from build123d import *

# Parameters (mm, degrees)
BOSS_EXTRUDE1_DEPTH = 1.016


with BuildPart() as part:
    # Sketch1 → Boss-Extrude1 (new body)
    with BuildSketch(Plane.XY):
        with BuildLine():
            Line((-102.690520384, 151.318398839), (-130.138661403, 140.228630017))
            ThreePointArc((-130.138661403, 140.228630017), (-139.028894565, 132.36321613), (-140.988038021, 120.655836484))
            Line((-140.988038021, 120.655836484), (-122.083041186, 13.440271634))
            ThreePointArc((-122.083041186, 13.440271634), (-118.354836941, 5.294136523), (-111.127725304, 0))
            Line((-111.127725304, 0), (111.127725304, 0))
            ThreePointArc((111.127725304, 0), (118.354836941, 5.294136523), (122.083041186, 13.440271634))
            Line((122.083041186, 13.440271634), (140.988038021, 120.655836484))
            ThreePointArc((140.988038021, 120.655836484), (139.028894565, 132.36321613), (130.138661403, 140.228630017))
            Line((130.138661403, 140.228630017), (102.690520384, 151.318398839))
            ThreePointArc((102.690520384, 151.318398839), (92.216863272, 163.055161588), (95.154949405, 178.50885833))
            ThreePointArc((95.154949405, 178.50885833), (122.006673364, 200.829543277), (155.995276019, 208.829727371))
            Line((155.995276019, 208.829727371), (246.294572316, 208.829727371))
            ThreePointArc((246.294572316, 208.829727371), (251.682725989, 211.061573699), (253.914572316, 216.449727371))
            Line((253.914572316, 216.449727371), (253.914572316, 220.98))
            ThreePointArc((253.914572316, 220.98), (251.682725989, 226.368153673), (246.294572316, 228.6))
            Line((246.294572316, 228.6), (47.442005026, 228.6))
            ThreePointArc((47.442005026, 228.6), (20.63063365, 239.70563365), (9.525, 266.517005026))
            Line((9.525, 266.517005026), (9.525, 609.6))
            Line((9.525, 609.6), (-9.525, 609.6))
            Line((-9.525, 609.6), (-9.525, 266.517005026))
            ThreePointArc((-9.525, 266.517005026), (-20.63063365, 239.70563365), (-47.442005026, 228.6))
            Line((-47.442005026, 228.6), (-551.265427684, 228.6))
            ThreePointArc((-551.265427684, 228.6), (-556.653581357, 226.368153673), (-558.885427684, 220.98))
            Line((-558.885427684, 220.98), (-558.885427684, 216.449727371))
            ThreePointArc((-558.885427684, 216.449727371), (-556.653581357, 211.061573699), (-551.265427684, 208.829727371))
            Line((-551.265427684, 208.829727371), (-155.995276019, 208.829727371))
            ThreePointArc((-155.995276019, 208.829727371), (-122.006673364, 200.829543277), (-95.154949405, 178.50885833))
            ThreePointArc((-95.154949405, 178.50885833), (-92.216863272, 163.055161588), (-102.690520384, 151.318398839))
        make_face()
    extrude(amount=BOSS_EXTRUDE1_DEPTH)


solid = part.part
Verification items for the finished model (mm, model axes). A direction names the side the tool comes from. Coordinates: 2 decimals unless noted, no trailing zeros. Order: outer loops, then holes, each group sorted by start corner. A loop starts at its lowest first (then second) coordinate and runs counter-clockwise, first axis right, second up.
1. Release check for a two-part mould opening along Y. For faces 3 (the face through (131.403, 66.298, 0.501)), 4 (the face through (20.93, 239.41, 0.5)), 5 (the face through (-34, 171, 1.016)), 6 (the face through (-122.45, 201.05, 0.5)) record: +Y half, -Y half, draft (parallel to the pull), parting line (faces both ways), or undercut.
Results found:
face 3: -Y half
face 4: +Y half
face 5: draft
face 6: undercut
2. Sectioned sample at A-A, the plane z = 0.25. Record the cut outline in (x, y) (3 decimals), and give its area (3 significant figures).
Results found:
outline: (-558.885, 216.45) arc R7.62 ccw to (-551.265, 208.83) - (-155.995, 208.83) arc R76.2 cw to (-95.155, 178.509) arc R17.78 cw to (-102.691, 151.318) - (-130.139, 140.229) arc R17.78 ccw to (-140.988, 120.656) - (-122.083, 13.44) arc R17.78 ccw to (-111.128, 0) - (111.128, 0) arc R17.78 ccw to (122.083, 13.44) - (140.988, 120.656) arc R17.78 ccw to (130.139, 140.229) - (102.691, 151.318) arc R17.78 cw to (95.155, 178.509) arc R76.2 cw to (155.995, 208.83) - (246.295, 208.83) arc R7.62 ccw to (253.915, 216.45) - (253.915, 220.98) arc R7.62 ccw to (246.295, 228.6) - (47.442, 228.6) arc R37.917 cw to (9.525, 266.517) - (9.525, 609.6) - (-9.525, 609.6) - (-9.525, 266.517) arc R37.917 cw to (-47.442, 228.6) - (-551.265, 228.6) arc R7.62 ccw to (-558.885, 220.98) - close
area: 75,300 mm2
3. Go/stop test with a flat-tipped pin: pin 1 Ø0.5 at (x, z) = (202.5, 0.5) entering from -Y. Record where the tip stops, or that it passes through.
Results found:
pin 1: stops at y = 208.83
4. Sectioned sample at C-C, the plane y = 458.5. Record the cut outline in (x, z) (3 decimals).
Results found:
outline: (-9.525, 0) - (9.525, 0) - (9.525, 1.016) - (-9.525, 1.016) - close
5. Scan lines: line 1 (Y direction, x = -292.5, z = 0.85); line 2 (X direction, y = 380.5, z = 0.35) (3 decimals); line 3 (Y direction, x = -89.5, z = 0.25). Record each from-to range of solid material in increasing order.
Results found:
line 1: y = 208.83 to 228.6
line 2: x = -9.525 to 9.525
line 3: y = 0 to 228.6
6. Sectioned sample at B-B, the plane x = -249. Record the cut outline in (y, z), and give its area (3 significant figures).
Results found:
outline: (208.83, 0) - (228.6, 0) - (228.6, 1.02) - (208.83, 1.02) - close
area: 20.1 mm2
7. Set-up check for faces 1 (the face through (121.57, 200.61, 0.5)), 2 (the face through (-34, 171, 0)): record each of +Z, -Z, +X, -X, +Y, -Y from which the full face is reachable in a straight line by a thin tool's end or side.
Results found:
face 1: +Z, -Z, +X
face 2: -Z, +X, -X, +Y, -Y
